Autodesk Inventor part; units mm, degrees
ref_plane "YZ Plane" through (0, 0, 0) normal (1, 0, 0) x (0, 1, 0)
ref_plane "XZ Plane" through (0, 0, 0) normal (0, 1, 0) x (-1, 0, 0)
ref_plane "XY Plane" through (0, 0, 0) normal (0, 0, 1) x (1, 0, 0)
sketch "Sketch1" plane through (0, 0, 0) normal (0, 1, 0) x (-1, 0, 0)
  circle A0 centre (0, 0) radius 19.2963
  circle A1 centre (0, 0) radius 20.2963
  dimension "d0" = 38.5926
  dimension "d7" = 40.5926
extrude "Extrusion2" add sketch "Sketch1" along normal blind 12.59
sketch "Sketch2" plane through (0, 12.59, 0) normal (0, 1, 0) x (1, 0, 0)
  circle A0 centre (0, 0) radius 19.2963
  circle A1 centre (0, 0) radius 18.2963
  dimension "d12" = 38.5926
  dimension "d13" = 36.5926
extrude "Extrusion3" add sketch "Sketch2" against normal blind 3.1
sketch "Sketch3" plane through (0, 0, 0) normal (0, -1, 0) x (1, 0, 0)
  circle A0 centre (0, 0) radius 19.2963
  circle A1 centre (0, 0) radius 18.2963
  dimension "d16" = 38.5926
  dimension "d17" = 36.5926
extrude "Extrusion4" add sketch "Sketch3" against normal blind 3.1
equation "\"d7\" = -2 * WoodThickness + 2 * d176 - 2 * d125"
equation "\"d12\" = d0"
equation "\"d16\" = d0"
equation "\"WoodThickness\" = 6.39"
equation "\"BearingHolderHeight\" = 13.1"
properties part number "CouplingHead_Silicone" material "UHMW, White"
Source: CAD feature listing. Evaluate the final solid. Frame: model axes, mm. A direction names the side the tool comes from. Give positions to 0.01 mm unless a question says otherwise; leave off trailing zeros. Write each loop counter-clockwise with the first axis right and the second up, starting at its lowest first coordinate (ties: lowest second). Pieces come first, ordered by that corner, then holes. Notation, with made-up numbers: M 9,20.25 L 24,20.25 A24 cw 24,53.25 Z; hole C 44.25,-20.5 d4. An arc over 180 degrees is marked long. Answer as a JSON object with one key per item and string values.
Q1. Cut plane A-A, the plane x = 0. Return the cut outline in (y, z), then the cut area to 3 significant figures.
Geometry check:
{"outline": "M 0,-20.3 L 12.59,-20.3 L 12.59,-18.3 L 9.49,-18.3 L 9.49,-19.3 L 3.1,-19.3 L 3.1,-18.3 L 0,-18.3 Z; M 0,18.3 L 3.1,18.3 L 3.1,19.3 L 9.49,19.3 L 9.49,18.3 L 12.59,18.3 L 12.59,20.3 L 0,20.3 Z", "area": "37.6 mm^2"}
Q2. Cut plane B-B, the plane z = -9.5. Return the cut outline in (x, y).
Geometry check:
{"outline": "M -17.94,0 L -15.64,0 L -15.64,3.1 L -16.8,3.1 L -16.8,9.49 L -15.64,9.49 L -15.64,12.59 L -17.94,12.59 Z; M 15.64,0 L 17.94,0 L 17.94,12.59 L 15.64,12.59 L 15.64,9.49 L 16.8,9.49 L 16.8,3.1 L 15.64,3.1 Z"}
Q3. Ray query, line 1 along Z through (x, y) = (0, 0.95); line 2 along Y through (x, z) = (-13, -13.5); line 3 along Z through (x, y) = (0, 5.25). Return the intervals inside material, ascending.
Geometry check:
{"line 1": "z = -20.3 to -18.3, 18.3 to 20.3", "line 2": "y = 0 to 3.1, 9.49 to 12.59", "line 3": "z = -20.3 to -19.3, 19.3 to 20.3"}
Q4. Cut plane C-C, the plane y = 5.25. Return the cut outline in (x, z).
Geometry check:
{"outline": "C 0,0 d40.59; hole C 0,0 d38.59"}
Q5. Contact query for flat-ended pins moving along their axis: P1, Ø2, axis at y = 7.5, z = 2, coming from the +X side; P2, Ø1, axis at x = 13, y = 4.5, coming from the -Z side; P3, Ø2, axis at x = 7, y = 10.5, coming from the +Z side. Output: stop coordinate, or through.
Geometry check:
{"P1": "stops at x = 20.27", "P2": "stops at z = -15.99", "P3": "stops at z = 19.39"}
Q6. Mould query, pull axis Y, two halves, no side actions, for faces 1 (the face through (-11, 0, 15)), 2 (the face through (19.278, 6.25, -0.848)), 3 (the face through (-14.52, 11.06, 11.13)), 4 (the face through (11, 12.59, 15)). Classes: +Y half, -Y half, draft (parallel to the pull), parting line (faces both ways), or undercut.
Geometry check:
{"face 1": "-Y half", "face 2": "undercut", "face 3": "draft", "face 4": "+Y half"}
Q7. Access query for faces 5 (the face through (16.106, 6.207, 12.35)), 6 (the face through (7.1, 3.1, -17.1)). Directions: +Z, -Z, +X, -X, +Y, -Y. A direction counts if a zero-diameter tool reaches every point of the face in a straight line with its end or side. Return the directions, or none.
Geometry check:
{"face 5": "+Y, -Y", "face 6": "none"}
